CAD build for the part. Positions are in the model's coordinates, mm. A direction names the side the tool comes from. Coordinates: 2 decimals unless noted, no trailing zeros. Loops run counter-clockwise (first coordinate to the right, second up) from the corner with the lowest first, then second, coordinate; pieces in that order, holes last. Notation, with made-up numbers: (61.25, 37.25) -> (74.25, 37.25) arc R24 cw to (74.25, 50.25) -> close; hole circle Ø5 at (65, 88). An arc over 180 degrees is marked (long way). Answer as a JSON object with one key per item and string values. Group by question number.
from build123d import *

# Parameters (mm, degrees)
BOSS_EXTRUDE1_DEPTH  = 3.6068
SKETCH2_W            = 4.5593
SKETCH2_H            = 2.032
M7_CLEARANCE_HOLE1_D = 7.9502


with BuildPart() as part:
    # Sketch1 → Boss-Extrude1 (new body)
    with BuildSketch(Plane.XY.offset(3.6068)):
        with BuildLine():
            Line((102.341394541, 120.371267572), (121.498125987, 120.371267572))
            ThreePointArc((121.498125987, 120.371267572), (124.416560264, 128.471327572), (121.498125987, 136.571387572))
            Line((121.498125987, 136.571387572), (102.341394541, 136.571387572))
            ThreePointArc((102.341394541, 136.571387572), (99.422960264, 128.471327572), (102.341394541, 120.371267572))
        make_face()
    extrude(amount=-BOSS_EXTRUDE1_DEPTH)

    # Sketch2 → Revolve1 (revolve)
    with BuildSketch(Plane.XZ.offset(-128.471327572), mode=Mode.PRIVATE) as revolve1_sk:
        with Locations((119.558810264, 4.6228)):
            Rectangle(SKETCH2_W, SKETCH2_H)
    revolve(revolve1_sk.sketch.rotate(Axis((117.279160264, 128.471327572, 5.6388), (0, 0, -1)), 180), axis=Axis((117.279160264, 128.471327572, 5.6388), (0, 0, -1)))

    # M7 Clearance Hole1 (through all)
    with Locations(Plane(origin=(0, 0, 0), x_dir=(-1, 0, 0), z_dir=(0, 0, -1))):
        with Locations((-117.279160264, 128.471327572)):
            Hole(M7_CLEARANCE_HOLE1_D / 2)


solid = part.part
Item 1: Band-saw the part on B-B, the plane x = 114.75. List the corners of the cut face in (y, z).
Item 2: Pull direction X, two halves, no side cores. Call faces 3 (the flat face through (112, 129, 0)), 4 (the cylindrical face through (114.35, 131.16, 2.86)), 5 (the cylindrical face through (124.416, 128.348, 1.829)): +X half, -X half, draft (parallel to the pull), parting line (faces both ways), or undercut.
Item 3: Flat gauge pins, fed straight in: P1, Ø5, axis at x = 117.28, y = 128.47, coming from the +Z side; P2, Ø1.5, axis at x = 116, z = 5, coming from the -Y side; P3, Ø3, axis at y = 131, z = 1.5, coming from the +X side. Where does each tip first touch, or does it go through?
Item 4: Band-saw the part on C-C, the plane z = 0.95. List the corners of the cut face in (x, y), and give its area (3 significant figures).
Item 5: 3-axis set-ups, long thin cutter, end or side, ignore diameter. For faces 1 (the cylindrical face through (114.8, 132.3, 4.6)), 2 (the flat face through (112, 120.371, 2)): which of +Z, -Z, +X, -X, +Y, -Y reach the whole face in a straight line?
Item 6: Band-saw the part on A-A, the plane y = 129.5. List the corners of the cut face in (x, z), and give its area (3 significant figures).
Item 7: Drill centre lines: L1, parallel to Z at x = 108.25, y = 134.5; L2, parallel to X at y = 128.25, z = 0.4; L3, parallel to Y at x = 115.5, z = 1.55. Where is each one in solid material? Low to high.
Item 8: Band-saw the part on D-D, the plane x = 103.5. List the corners of the cut face in (y, z).
Reply:
{
 "1": {"outline": "(120.37, 0) -> (125.4, 0) -> (125.4, 5.64) -> (124.68, 5.64) -> (124.68, 3.61) -> (120.37, 3.61) -> close; (131.54, 0) -> (136.57, 0) -> (136.57, 3.61) -> (132.26, 3.61) -> (132.26, 5.64) -> (131.54, 5.64) -> close"},
 "2": {"face 3": "draft", "face 4": "undercut", "face 5": "+X half"},
 "3": {"P1": "through", "P2": "y = 123.94", "P3": "x = 124.37"},
 "4": {"outline": "(102.34, 120.37) -> (121.5, 120.37) arc R12.7 ccw to (121.5, 136.57) -> (102.34, 136.57) arc R12.7 ccw to start; hole circle Ø7.95 at (117.28, 128.47)", "area": "325 mm²"},
 "5": {"face 1": "+Z", "face 2": "+Z, -Z, +X, -X, -Y"},
 "6": {"outline": "(99.46, 0) -> (113.44, 0) -> (113.44, 5.64) -> (112.84, 5.64) -> (112.84, 3.61) -> (99.46, 3.61) -> close; (121.12, 0) -> (124.37, 0) -> (124.37, 3.61) -> (121.72, 3.61) -> (121.72, 5.64) -> (121.12, 5.64) -> close", "area": "64.6 mm²"},
 "7": {"L1": "0 to 3.61", "L2": "99.42 to 113.31, 121.25 to 124.41", "L3": "120.37 to 124.92, 132.03 to 136.57"},
 "8": {"outline": "(120.37, 0) -> (136.57, 0) -> (136.57, 3.61) -> (120.37, 3.61) -> close"}
}
